Check sheet for the modelled part. Datum: model origin and axes. Units: mm. A direction names the side the tool comes from. Give positions to 0.01 mm unless a question says otherwise; leave off trailing zeros. Loops run counter-clockwise (first coordinate to the right, second up) from the corner with the lowest first, then second, coordinate; pieces in that order, holes last. Notation, with made-up numbers: M 65.25,59 L 116.25,59 A33 cw 116.25,87 Z; hole C 46,-28 d2. An arc over 180 degrees is marked long. Use one line per item in the form item = value.
Autodesk Inventor part; units mm, degrees
ref_plane "YZ Plane" through (0, 0, 0) normal (1, 0, 0) x (0, 1, 0)
ref_plane "XZ Plane" through (0, 0, 0) normal (0, 1, 0) x (-1, 0, 0)
ref_plane "XY Plane" through (0, 0, 0) normal (0, 0, 1) x (1, 0, 0)
sketch "Sketch1" plane through (0, 0, 0) normal (1, 0, 0) x (0, 1, 0)
  line L0 (31.75, 82.55) -> (-31.75, 82.55)
  line L1 (-31.75, 82.55) -> (-31.75, -82.55)
  line L2 (-31.75, -82.55) -> (31.75, -82.55)
  line L3 (31.75, -82.55) -> (31.75, 82.55)
  point P0 (0, 0)
  point P1 (31.75, 0)
  point P2 (0, 82.55)
  dimension "d0" = 165.1
  dimension "d1" = 63.5
extrude "Extrusion1" add sketch "Sketch1" along normal blind 12.7
sketch "Sketch3" plane through (12.7, 0, 0) normal (1, 0, 0) x (0, 0, -1)
  line L0 (72.898, -22.098) -> (-72.898, -22.098)
  line L1 (-72.898, -22.098) -> (-72.898, 22.098)
  line L2 (-72.898, 22.098) -> (72.898, 22.098)
  line L3 (72.898, 22.098) -> (72.898, -22.098)
  line L4 (72.898, -22.098) -> (-72.898, 22.098) construction
  line L5 (-72.898, -22.098) -> (72.898, 22.098) construction
  line L6 (79.375, -28.575) -> (-79.375, -28.575)
  line L7 (-79.375, -28.575) -> (-79.375, 28.575)
  line L8 (-79.375, 28.575) -> (79.375, 28.575)
  line L9 (79.375, 28.575) -> (79.375, -28.575)
  line L10 (79.375, -28.575) -> (-79.375, 28.575) construction
  line L11 (-79.375, -28.575) -> (79.375, 28.575) construction
  point P0 (0, 0)
  point P1 (0, 0)
  point P2 (0, 0)
  dimension "d16" = 145.796
  dimension "d17" = 44.196
  dimension "d18" = 6.477
  dimension "d19" = 6.477
extrude "Extrusion3" cut sketch "Sketch3" against normal blind 3.175
fillet "Fillet1" radius 3.175 8 edges at (11.1125, -28.575, 79.375) (11.1125, 28.575, 79.375) (11.1125, 28.575, -79.375) (11.1125, -28.575, -79.375) (11.1125, -22.098, 72.898) (11.1125, 22.098, 72.898) (11.1125, 22.098, -72.898) (11.1125, -22.098, -72.898)
sketch "Sketch4" plane through (0, 0, 0) normal (-1, 0, 0) x (0, 0, 1)
  line L0 (0, 0) -> (27.5167, 0) construction
  line L1 (82.55, 31.75) -> (82.55, -31.75)
  dimension "d42" = 55.0333
hole "Hole1" at (0, 0, 27.5167) direction (1, 0, 0) diameter 13.0969 end through all
sketch "Sketch5" plane through (0, 0, 0) normal (-1, 0, 0) x (0, 0, 1)
  circle A0 centre (27.5167, 0) radius 6.5484
  line L0 (42.7567, 10.795) -> (12.2767, 10.795) construction
  line L1 (12.2767, 10.795) -> (12.2767, -10.795) construction
  line L2 (12.2767, -10.795) -> (42.7567, -10.795) construction
  line L3 (42.7567, -10.795) -> (42.7567, 10.795) construction
  line L4 (42.7567, 10.795) -> (12.2767, -10.795) construction
  line L5 (12.2767, 10.795) -> (42.7567, -10.795) construction
  point P0 (0, 0)
  dimension "d30" = 30.48
  dimension "d31" = 21.59
hole "Hole2" at (0, -10.795, 42.7567) at (0, 10.795, 42.7567) at (0, 10.795, 12.2767) at (0, -10.795, 12.2767) direction (1, 0, 0) diameter 2.159 depth 8.8646 tip angle 118
pattern_linear "Rectangular Pattern1" count 2 spacing 55.0333 along (0, 0, -1) of "Hole1", "Hole2"
equation "\"d0\" = tubeWidth + 2 * plateOverhang"
equation "\"d1\" = tubeHeight + 2 * plateOverhang"
equation "\"d2\" = sensorCapThickness"
equation "\"d16\" = -2 * tubeWallThickness + tubeWidth - 2 * tubePlateClearance"
equation "\"d17\" = -2 * tubeWallThickness + tubeHeight - 2 * tubePlateClearance"
equation "\"d18\" = tubeWallThickness + tubePlateClearance + moatWidth"
equation "\"d19\" = tubeWallThickness + tubePlateClearance + moatWidth"
equation "\"d12\" = moatDepth"
equation "\"d23\" = glassTubeDiameter + 2 * glassTubeClearance"
equation "\"d30\" = longHoleSpacing"
equation "\"d31\" = shortHoleSpacing"
equation "\"tubeHeight\" = 50.8"
equation "\"tubeWidth\" = 152.4"
equation "\"tubeLength\" = 304.8"
equation "\"tubeWallThickness\" = 3.175"
equation "\"plateOverhang\" = 6.35"
equation "\"moatWidth\" = 3.175"
equation "\"tubePlateClearance\" = 0.127"
equation "\"moatDepth\" = 3.175"
equation "\"blankCapThickness\" = 9.525"
equation "\"sensorCapThickness\" = 12.7"
equation "\"glassTubeDiameter\" = 12.7"
equation "\"glassTubeClearance\" = 0.19844"
equation "\"shortHoleSpacing\" = 21.59"
equation "\"longHoleSpacing\" = 30.48"
equation "\"oRingGrooveWidth\" = 2.54"
equation "\"oRingGrooveDepth\" = 1.2446"
equation "\"fiberDiameter\" = 1"
equation "\"sensorHolderDiameter\" = 50.8"
equation "\"oRingID\" = 22.2504"
equation "\"sensorHolderThickness\" = 12.7"
equation "\"fiberClearance\" = 0"
equation "\"glassTubeLength\" = 279.4"
equation "\"glassTubeID\" = 7.874"
equation "\"sensorBoardHoleSpacing\" = 19"
properties part number "plateEnd" material "Aluminum 6061"
1) Section check D-D (y = -27). Record the cut outline in (x, z) (3 decimals), then the cut area to 3 significant figures.
Evaluation:
outline = M 0,-82.55 L 12.7,-82.55 L 12.7,-78.942 L 9.525,-78.942 L 9.525,78.942 L 12.7,78.942 L 12.7,82.55 L 0,82.55 Z
area = 1,600 mm^2
2) Scan lines: line 1 (Y direction, x = 10, z = 68.5) (3 decimals); line 2 (Z direction, x = 8.5, y = 0); line 3 (Z direction, x = 4.5, y = 11). Record each from-to range of solid material in increasing order.
Evaluation:
line_1 = -31.75 to -28.575, -22.098 to 22.098, 28.575 to 31.75
line_2 = -82.55 to -34.07, -20.97 to 20.97, 34.07 to 82.55
line_3 = -82.55 to -43.82, -41.7 to -13.34, -11.22 to 11.22, 13.34 to 41.7, 43.82 to 82.55
3) Section check A-A (y = 0). Record the cut outline in (x, z) (3 decimals), then the cut area to 3 significant figures.
Evaluation:
outline = M 0,-82.55 L 12.7,-82.55 L 12.7,-79.375 L 9.525,-79.375 L 9.525,-72.898 L 12.7,-72.898 L 12.7,-34.065 L 0,-34.065 Z; M 0,-20.968 L 12.7,-20.968 L 12.7,20.968 L 0,20.968 Z; M 0,34.065 L 12.7,34.065 L 12.7,72.898 L 9.525,72.898 L 9.525,79.375 L 12.7,79.375 L 12.7,82.55 L 0,82.55 Z
area = 1,720 mm^2
4) Set-up check for faces 1 (the face through (0, 0, 1)), 2 (the face through (11.09, -27.67, 78.42)): record each of +Z, -Z, +X, -X, +Y, -Y from which the full face is reachable in a straight line by a thin tool's end or side.
Evaluation:
face_1 = +Z, -Z, -X, +Y, -Y
face_2 = +X
5) Release check for a two-part mould opening along Z. For faces 3 (the face through (6, 0, -82.55)), 4 (the face through (6, 31.75, -1)), 5 (the face through (11, 28.575, 1)) record: pulls with the +Z half, pulls with the -Z half, needs draft (parallel to the pull), parting line crosses it, or undercut.
Evaluation:
face_3 = pulls with the -Z half
face_4 = needs draft
face_5 = undercut
6) Depth check by flat-ended pin: pin 1 Ø1.7 at (y, z) = (-10.8, -12.28) entering from -X; pin 2 Ø1.9 at (y, z) = (10.8, 42.76) entering from -X. Enter the tip coordinate at first touch or a pass-through.
Evaluation:
pin_1 = 9
pin_2 = 8.94
7) Section check B-B (z = 56). Record the cut outline in (x, y) (3 decimals), then the cut area to 3 significant figures.
Evaluation:
outline = M 0,-31.75 L 12.7,-31.75 L 12.7,-28.575 L 9.525,-28.575 L 9.525,-22.098 L 12.7,-22.098 L 12.7,22.098 L 9.525,22.098 L 9.525,28.575 L 12.7,28.575 L 12.7,31.75 L 0,31.75 Z
area = 765 mm^2
8) Section check C-C (x = 7). State how many separate pieces and enclosed holes the cut face has, then the cut area to 3 significant figures.
Evaluation:
separate_pieces = 1
enclosed_holes = 10
area = 10,200 mm^2
